Work out the finished part from the listing and answer in its coordinate system (mm). A direction names the side the tool comes from. Coordinates: 2 decimals unless noted, no trailing zeros. Order: outer loops, then holes, each group sorted by start corner. A loop starts at its lowest first (then second) coordinate and runs counter-clockwise, first axis right, second up. Notation, with made-up numbers: M 70,53 L 105,53 A15 ccw 105,78 Z; hole C 42,9 d3. An arc over 180 degrees is marked long. Answer in a Markdown table with one row per item. Add a question column.
Item 1: The mould has two halves that part along X. Classify faces 3 (the face through (47.5, 0, 1)), 4 (the face through (0, 0, 0)), 5 (the face through (-24.75, 15.12, 1.48)): released by +X, released by -X, zero draft, split by the parting line, or undercut.
Item 2: Which of the six approach directions +Z, -Z, +X, -X, +Y, -Y give full straight-line access (tool end or side, diameter ignored) to faces 1 (the face through (10.65, -3.36, 1.48)), 2 (the face through (46.074, 32.221, 1.479))?
Item 3: The part is cut by section B-B (x = 24.5). Write down the section's boundary in (y, z) (3 decimals), then the cut area to 3 significant figures.
Item 4: The part is cut by section D-D (z = 0.6). State how many separate pieces and enclosed holes the cut face has, then the cut area to 3 significant figures.
Item 5: The part is cut by section A-A (y = -9.5). Write down the section's boundary in (x, z).
Item 6: Consider line 1 (Y direction, x = -42.5, z = 2.15) (3 decimals); line 2 (X direction, y = 4, z = 0.85); line 3 (X direction, y = 25.5, z = 0.2). Determine where each line is inside the solid, lowest interval first. Write a range as from..to.
Item 7: The part is cut by section C-C (x = 9.5). Write down the section's boundary in (y, z) (3 decimals).
from build123d import *

# Parameters (mm, degrees)
SKETCH_1_R      = 5
SKETCH_1_R_2    = 1.55
EXTRUDE_1_DEPTH = 3
FILLET_1_R      = 2
FILLET_2_R      = 1


with BuildPart() as part:
    # 草图1 → 凸台-拉伸1 (new body)
    # profile 1 of 5: a face of its own
    with BuildSketch(Plane.XY):
        with BuildLine():
            Line((-42.5, -33.725), (42.5, -33.725))
            ThreePointArc((42.5, -33.725), (39.761387212, -32.908300133), (37.917424305, -30.725))
            Line((37.917424305, -30.725), (2, -30.725))
            Line((2, -30.725), (2, -3.872835094))
            Line((2, -3.872835094), (37.513133211, -29.087159674))
            ThreePointArc((37.513133211, -29.087159674), (37.811061724, -26.988953387), (38.951354438, -25.202626557))
            Line((38.951354438, -25.202626557), (6.271598724, -2))
            Line((6.271598724, -2), (44.5, -2))
            Line((44.5, -2), (44.5, -24.142424305))
            ThreePointArc((44.5, -24.142424305), (46.683300133, -25.986387212), (47.5, -28.725))
            Line((47.5, -28.725), (47.5, 28.725))
            ThreePointArc((47.5, 28.725), (46.683300133, 25.986387212), (44.5, 24.142424305))
            Line((44.5, 24.142424305), (44.5, 2))
            Line((44.5, 2), (6.271598724, 2))
            Line((6.271598724, 2), (38.951354438, 25.202626557))
            ThreePointArc((38.951354438, 25.202626557), (37.811061724, 26.988953387), (37.513133211, 29.087159674))
            Line((37.513133211, 29.087159674), (2, 3.872835094))
            Line((2, 3.872835094), (2, 30.725))
            Line((2, 30.725), (37.917424305, 30.725))
            ThreePointArc((37.917424305, 30.725), (39.761387212, 32.908300133), (42.5, 33.725))
            Line((42.5, 33.725), (-42.5, 33.725))
            ThreePointArc((-42.5, 33.725), (-39.761387212, 32.908300133), (-37.917424305, 30.725))
            Line((-37.917424305, 30.725), (-2, 30.725))
            Line((-2, 30.725), (-2, 3.872835094))
            Line((-2, 3.872835094), (-37.513133211, 29.087159674))
            ThreePointArc((-37.513133211, 29.087159674), (-37.503284381, 28.906198862), (-37.5, 28.725))
            ThreePointArc((-37.5, 28.725), (-37.87705571, 26.820167699), (-38.951354438, 25.202626557))
            Line((-38.951354438, 25.202626557), (-6.271598724, 2))
            Line((-6.271598724, 2), (-44.5, 2))
            Line((-44.5, 2), (-44.5, 24.142424305))
            ThreePointArc((-44.5, 24.142424305), (-46.683300133, 25.986387212), (-47.5, 28.725))
            Line((-47.5, 28.725), (-47.5, -28.725))
            ThreePointArc((-47.5, -28.725), (-46.683300133, -25.986387212), (-44.5, -24.142424305))
            Line((-44.5, -24.142424305), (-44.5, -2))
            Line((-44.5, -2), (-6.271598724, -2))
            Line((-6.271598724, -2), (-38.951354438, -25.202626557))
            ThreePointArc((-38.951354438, -25.202626557), (-37.87705571, -26.820167699), (-37.5, -28.725))
            ThreePointArc((-37.5, -28.725), (-37.503284381, -28.906198862), (-37.513133211, -29.087159674))
            Line((-37.513133211, -29.087159674), (-2, -3.872835094))
            Line((-2, -3.872835094), (-2, -30.725))
            Line((-2, -30.725), (-37.917424305, -30.725))
            ThreePointArc((-37.917424305, -30.725), (-39.761387212, -32.908300133), (-42.5, -33.725))
        make_face()
    # profile 2 of 5: a face of its own
    with BuildSketch(Plane.XY):
        with Locations((-42.5, 28.725)):
            Circle(SKETCH_1_R)
        with Locations((-42.5, 28.725)):
            Circle(SKETCH_1_R_2, mode=Mode.SUBTRACT)
    # profile 3 of 5: a face of its own
    with BuildSketch(Plane.XY):
        with Locations((42.5, 28.725)):
            Circle(SKETCH_1_R)
        with Locations((42.5, 28.725)):
            Circle(SKETCH_1_R_2, mode=Mode.SUBTRACT)
    # profile 4 of 5: a face of its own
    with BuildSketch(Plane.XY):
        with Locations((42.5, -28.725)):
            Circle(SKETCH_1_R)
        with Locations((42.5, -28.725)):
            Circle(SKETCH_1_R_2, mode=Mode.SUBTRACT)
    # profile 5 of 5: a face of its own
    with BuildSketch(Plane.XY):
        with Locations((-42.5, -28.725)):
            Circle(SKETCH_1_R)
        with Locations((-42.5, -28.725)):
            Circle(SKETCH_1_R_2, mode=Mode.SUBTRACT)
    extrude(amount=EXTRUDE_1_DEPTH)

    # 圆角1
    # the kernel refuses this fillet: 2 mm, written as the material it adds along each edge
    with BuildSketch(Plane(origin=(38.951354438, 25.202626557, 0), x_dir=(-0.8153829846202765, -0.5789219190803973, 0), z_dir=(0, 0, 1)), Plane(origin=(-38.951354438, -25.202626557, 0), x_dir=(0.8153829846202759, 0.5789219190803978, 0), z_dir=(0, 0, 1))) as fillet_1_piece_1:
        with BuildLine():
            CenterArc((1.475169897, 2), FILLET_1_R, 203.736299512, 66.263700488)
            ThreePointArc((-0.355645617, 1.194944379), (-0.140432135, 0.608600598), (0, 0))
            Line((0, 0), (1.475169897, 0))
        make_face()
    extrude(amount=3)
    with BuildSketch(Plane(origin=(6.271598724, 2, 0), x_dir=(1, 0, 0), z_dir=(0, 0, 1)), Plane(origin=(6.271598724, -2, 0), x_dir=(0.8153829846202769, -0.5789219190803966, 0), z_dir=(0, 0, 1)), Plane(origin=(-6.271598724, -2, 0), x_dir=(-1, 0, 0), z_dir=(0, 0, 1)), Plane(origin=(-6.271598724, 2, 0), x_dir=(-0.8153829846202769, 0.5789219190803967, 0), z_dir=(0, 0, 1))) as fillet_1_piece_2:
        with BuildLine():
            CenterArc((FILLET_1_R * 3.13579936221, FILLET_1_R), FILLET_1_R, 125.374751844, 144.625248156)
            Line((FILLET_1_R * 2.55687744313, FILLET_1_R * 1.81538298462), (0, 0))
            Line((0, 0), (FILLET_1_R * 3.13579936221, 0))
        make_face()
    extrude(amount=3)
    with BuildSketch(Plane(origin=(44.5, 2, 0), x_dir=(0, 1, 0), z_dir=(0, 0, 1)), Plane(origin=(44.5, -2, 0), x_dir=(-1, 0, 0), z_dir=(0, 0, 1)), Plane(origin=(2, -30.725, 0), x_dir=(1, 0, 0), z_dir=(0, 0, 1)), Plane(origin=(-2, -30.725, 0), x_dir=(0, 1, 0), z_dir=(0, 0, 1)), Plane(origin=(-44.5, -2, 0), x_dir=(0, -1, 0), z_dir=(0, 0, 1)), Plane(origin=(-44.5, 2, 0), x_dir=(1, 0, 0), z_dir=(0, 0, 1)), Plane(origin=(-2, 30.725, 0), x_dir=(-1, 0, 0), z_dir=(0, 0, 1)), Plane(origin=(2, 30.725, 0), x_dir=(0, -1, 0), z_dir=(0, 0, 1))) as fillet_1_piece_3:
        with BuildLine():
            CenterArc((FILLET_1_R, FILLET_1_R), FILLET_1_R, 180, 90)
            Line((0, FILLET_1_R), (0, 0))
            Line((0, 0), (FILLET_1_R, 0))
        make_face()
    extrude(amount=3)
    with BuildSketch(Plane(origin=(44.5, 24.142424305, 0), x_dir=(0, -1, 0), z_dir=(0, 0, 1)), Plane(origin=(37.917424305, -30.725, 0), x_dir=(-1, 0, 0), z_dir=(0, 0, 1)), Plane(origin=(-44.5, -24.142424305, 0), x_dir=(0, 1, 0), z_dir=(0, 0, 1)), Plane(origin=(-37.917424305, 30.725, 0), x_dir=(1, 0, 0), z_dir=(0, 0, 1))) as fillet_1_piece_4:
        with BuildLine():
            CenterArc((2.417424305, -2), FILLET_1_R, 90, 90)
            ThreePointArc((0.417424305, -2), (0.31195587, -0.978451782), (0, 0))
            Line((0, 0), (2.417424305, 0))
        make_face()
    extrude(amount=3)
    with BuildSketch(Plane(origin=(44.5, -24.142424305, 0), x_dir=(0, 1, 0), z_dir=(0, 0, 1)), Plane(origin=(-37.917424305, -30.725, 0), x_dir=(1, 0, 0), z_dir=(0, 0, 1)), Plane(origin=(-44.5, 24.142424305, 0), x_dir=(0, -1, 0), z_dir=(0, 0, 1)), Plane(origin=(37.917424305, 30.725, 0), x_dir=(-1, 0, 0), z_dir=(0, 0, 1))) as fillet_1_piece_5:
        with BuildLine():
            CenterArc((2.417424305, 2), FILLET_1_R, 180, 90)
            ThreePointArc((0.417424305, 2), (0.31195587, 0.978451782), (0, 0))
            Line((0, 0), (2.417424305, 0))
        make_face()
    extrude(amount=3)
    with BuildSketch(Plane(origin=(38.951354438, -25.202626557, 0), x_dir=(-0.8153829846202785, 0.5789219190803946, 0), z_dir=(0, 0, 1)), Plane(origin=(-38.951354438, 25.202626557, 0), x_dir=(0.8153829846202768, -0.5789219190803968, 0), z_dir=(0, 0, 1))) as fillet_1_piece_6:
        with BuildLine():
            CenterArc((1.475169897, -2), FILLET_1_R, 90, 66.263700488)
            ThreePointArc((-0.355645617, -1.194944379), (-0.140432135, -0.608600598), (0, 0))
            Line((0, 0), (1.475169897, 0))
        make_face()
    extrude(amount=3)
    with BuildSketch(Plane(origin=(2, -3.872835094, 0), x_dir=(0, -1, 0), z_dir=(0, 0, 1)), Plane(origin=(-2, -3.872835094, 0), x_dir=(-0.8153829846202767, -0.5789219190803968, 0), z_dir=(0, 0, 1)), Plane(origin=(-2, 3.872835094, 0), x_dir=(0, 1, 0), z_dir=(0, 0, 1)), Plane(origin=(2, 3.872835094, 0), x_dir=(0.8153829846202766, 0.578921919080397, 0), z_dir=(0, 0, 1))) as fillet_1_piece_7:
        with BuildLine():
            CenterArc((FILLET_1_R * 1.93641754717, FILLET_1_R), FILLET_1_R, 144.625248156, 125.374751844)
            Line((FILLET_1_R * 1.12103456255, FILLET_1_R * 1.57892191908), (0, 0))
            Line((0, 0), (FILLET_1_R * 1.93641754717, 0))
        make_face()
    extrude(amount=3)
    with BuildSketch(Plane(origin=(37.513133211, -29.087159674, 0), x_dir=(-0.8153829846202749, 0.5789219190803994, 0), z_dir=(0, 0, 1)), Plane(origin=(-37.513133211, 29.087159674, 0), x_dir=(0.8153829846202781, -0.5789219190803949, 0), z_dir=(0, 0, 1))) as fillet_1_piece_8:
        with BuildLine():
            CenterArc((0.849166367, 2), FILLET_1_R, 227.759477208, 42.240522792)
            ThreePointArc((-0.495322353, 0.519341335), (-0.23833117, 0.268569172), (0, 0))
            Line((0, 0), (0.849166367, 0))
        make_face()
    extrude(amount=3)
    with BuildSketch(Plane(origin=(-37.513133211, -29.087159674, 0), x_dir=(0.8153829846202739, 0.5789219190804008, 0), z_dir=(0, 0, 1)), Plane(origin=(37.513133211, 29.087159674, 0), x_dir=(-0.8153829846202756, -0.5789219190803985, 0), z_dir=(0, 0, 1))) as fillet_1_piece_9:
        with BuildLine():
            CenterArc((0.849166367, -2), FILLET_1_R, 90, 42.240522792)
            ThreePointArc((-0.495322353, -0.519341335), (-0.23833117, -0.268569172), (0, 0))
            Line((0, 0), (0.849166367, 0))
        make_face()
    extrude(amount=3)

    # 圆角2
    fillet_2_edges = [part.edges().sort_by_distance(p)[0] for p in [
        (-37.422632563, 29.275893843, 1.5),
        (-37.422632563, -29.275893843, 1.5),
        (37.422632563, -29.275893843, 1.5),
        (37.422632563, 29.275893843, 1.5),
    ]]
    fillet(fillet_2_edges, radius=FILLET_2_R)


solid = part.part
Reply:
| question | item | result |
|---|---|---|
| 1 | face 3 | released by +X |
| 1 | face 4 | zero draft |
| 1 | face 5 | undercut |
| 2 | face 1 | +Z, -Z |
| 2 | face 2 | +Z, -Z, +X, +Y |
| 3 | outline | M -33.725,0 L -30.725,0 L -30.725,3 L -33.725,3 Z; M -19.848,0 L -14.942,0 L -14.942,3 L -19.848,3 Z; M -2,0 L 2,0 L 2,3 L -2,3 Z; M 14.942,0 L 19.848,0 L 19.848,3 L 14.942,3 Z; M 30.725,0 L 33.725,0 L 33.725,3 L 30.725,3 Z |
| 3 | area | 59.4 mm2 |
| 4 | separate pieces | 1 |
| 4 | enclosed holes | 12 |
| 4 | area | 2,390 mm2 |
| 5 | outline | M -47.5,0 L -44.5,0 L -44.5,3 L -47.5,3 Z; M -16.83,0 L -9.93,0 L -9.93,3 L -16.83,3 Z; M -2,0 L 2,0 L 2,3 L -2,3 Z; M 9.93,0 L 16.83,0 L 16.83,3 L 9.93,3 Z; M 44.5,0 L 47.5,0 L 47.5,3 L 44.5,3 Z |
| 6 | line 1 | y = -33.725..-30.275, -27.175..-23.725, -2..2, 23.725..27.175, 30.275..33.725 |
| 6 | line 2 | x = -47.5..-44.5, -10.54..10.54, 44.5..47.5 |
| 6 | line 3 | x = -47.5..-32.46, -2..2, 32.46..47.5 |
| 7 | outline | M -33.725,0 L -30.725,0 L -30.725,3 L -33.725,3 Z; M -9.198,0 L 9.198,0 L 9.198,3 L -9.198,3 Z; M 30.725,0 L 33.725,0 L 33.725,3 L 30.725,3 Z |
